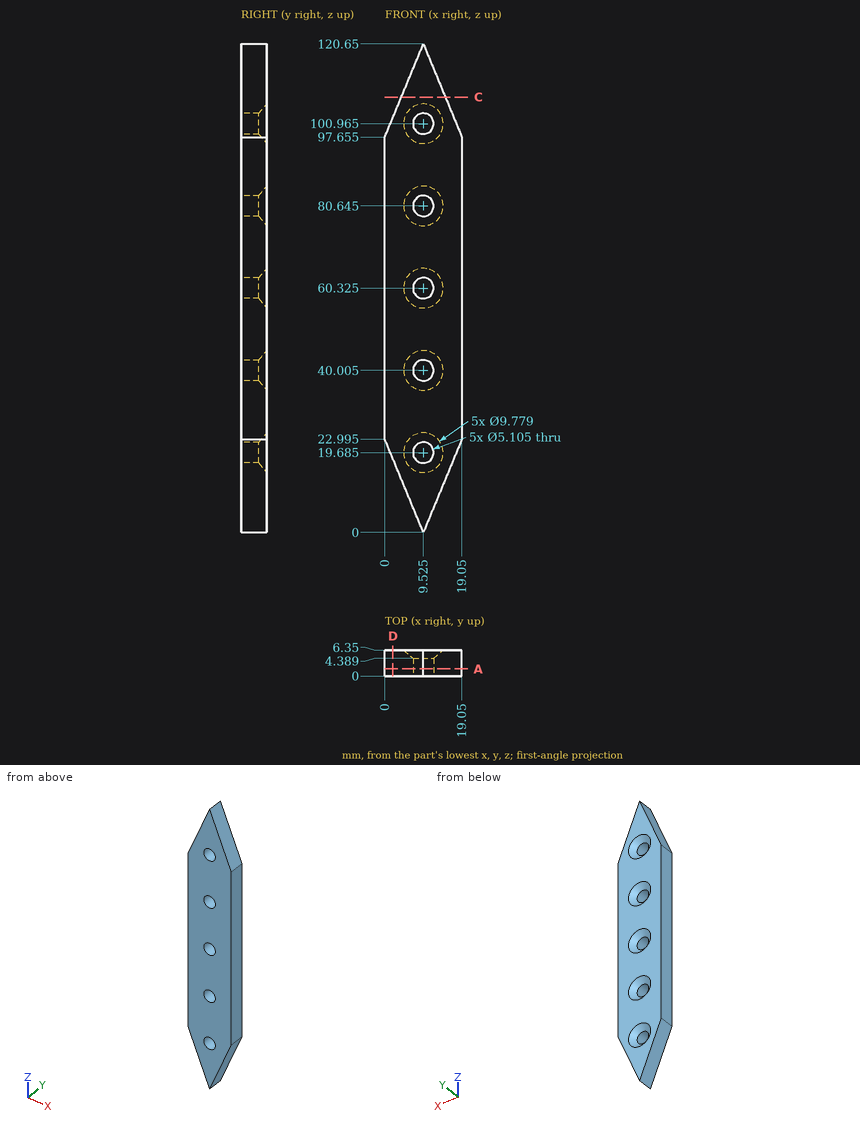
For this review, use the dimensioned drawing (mm, ordinates from the lowest corner) and the shaded views. Round coordinates to 2 decimals unless told otherwise and drop trailing zeros. Order: outer loops, then holes, each group sorted by start corner. A loop starts at its lowest first (then second) coordinate and runs counter-clockwise, first axis right, second up.
1) Clearance check with flat-ended pins moving along their axes: pin 1 Ø8 at (x, z) = (9.525, 80.645) entering from +Y (1 decimal); pin 2 Ø6.5 at (x, z) = (9.525, 100.965) entering from +Y (1 decimal); pin 3 Ø2 at (x, y) = (16.5, 2) entering from +Z (1 decimal); pin 4 Ø4 at (x, z) = (9.525, 40.005) entering from -Y. State where each tip first meets the part, or that it passes through.
The answers:
pin 1: stops at y = 5.6
pin 2: stops at y = 5
pin 3: stops at z = 106.2
pin 4: passes through
2) Consider section C-C (z = 107.5). State the section outline as (x, y) points.
The answers:
outline: (4.08, 0) - (14.97, 0) - (14.97, 6.35) - (4.08, 6.35) - close
3) Consider section A-A (y = 1.75). Count the separate pieces of the cut face and the enclosed holes in it, plus the area to 3 significant figures.
The answers:
separate pieces: 1
enclosed holes: 5
area: 1,760 mm2
4) Consider section D-D (x = 2). State the section outline as (y, z) points.
The answers:
outline: (0, 18.17) - (6.35, 18.17) - (6.35, 102.48) - (0, 102.48) - close
5) For L1, parallel to X at y = 0.5, z = 15; L2, parallel to Z at x = 1.5, y = 1.25 (1 decimal); L3, parallel to X at y = 1.75, z = 101.5, list the stretches that pass through material, from the lowest coordinate up.
The answers:
L1: x = 3.31 to 15.74
L2: z = 19.4 to 101.3
L3: x = 1.59 to 7.03, 12.02 to 17.46
